CAD build for the part. Positions are in the model's coordinates, mm. A direction names the side the tool comes from. Coordinates: 2 decimals unless noted, no trailing zeros. Order: outer loops, then holes, each group sorted by start corner. A loop starts at its lowest first (then second) coordinate and runs counter-clockwise, first axis right, second up. Notation, with made-up numbers: M 50.5,35 L 97.5,35 A23 ccw 97.5,70 Z; hole C 8.5,42 d11. An arc over 180 degrees is marked long. Write item = value, one per line.
Autodesk Inventor part; units mm, degrees
ref_plane "YZ Plane" through (0, 0, 0) normal (1, 0, 0) x (0, 1, 0)
ref_plane "XZ Plane" through (0, 0, 0) normal (0, 1, 0) x (-1, 0, 0)
ref_plane "XY Plane" through (0, 0, 0) normal (0, 0, 1) x (1, 0, 0)
sketch "Sketch1" plane through (0, 0, 0) normal (0, 0, 1) x (1, 0, 0)
  circle A0 centre (0, 0) radius 15
  dimension "d0" = 30
extrude "Extrusion1" add sketch "Sketch1" along normal blind 10
sketch "Sketch2" plane through (0, 0, 10) normal (0, 0, 1) x (1, 0, 0)
  circle A0 centre (0, 0) radius 15
  circle A1 centre (0, 0) radius 7.5
  dimension "d3" = 15
extrude "Extrusion2" add sketch "Sketch2" along normal blind 43.2 contours A1
sketch "Sketch3" plane through (0, 0, 53.2) normal (0, 0, 1) x (1, 0, 0)
  circle A0 centre (0, 0) radius 7.5
  circle A1 centre (0, 0) radius 6.5
  dimension "d6" = 1
extrude "Extrusion3" cut sketch "Sketch3" against normal blind 1 contours A1
fillet "Fillet1" radius 2 1 edges at (-15, 0, 10)
chamfer "Chamfer1" distance 0.25 angle 45 1 edges at (-7.5, 0, 53.2)
chamfer "Chamfer2" distance 0.25 angle 45 1 edges at (-15, 0, 0)
properties part number "InfiniStix_066x"
(1) Pull direction X, two halves, no side cores. Call faces 1 (the face through (-7.493, -0.33, 31.174)), 2 (the face through (-3, 6, 53.2)), 3 (the face through (-5.158, -3.955, 52.707)): +X half, -X half, draft (parallel to the pull), parting line (faces both ways), or undercut.
Evaluation:
face_1 = parting line
face_2 = draft
face_3 = undercut
(2) Pin check, flat tips, straight feed: pin 1 Ø6 at (x, z) = (9, 38) entering from +Y; pin 2 Ø10 at (x, z) = (-7, 22.5) entering from -Y; pin 3 Ø6 at (x, z) = (9.5, 34) entering from -Y; pin 4 Ø1.5 at (x, z) = (-8.5, 34) entering from +Y. Stop position of each tip, or through.
Evaluation:
pin_1 = 4.5
pin_2 = -7.23
pin_3 = -3.74
pin_4 = through
(3) Slice it at A-A, the plane x = 0. Write the cut outline in (y, z), then the cut area to 3 significant figures.
Evaluation:
outline = M -15,0.25 L -14.75,0 L 14.75,0 L 15,0.25 L 15,8 A2 ccw 13,10 L 7.5,10 L 7.5,52.95 L 7.25,53.2 L 6.5,53.2 L 6.5,52.2 L -6.5,52.2 L -6.5,53.2 L -7.25,53.2 L -7.5,52.95 L -7.5,10 L -13,10 A2 ccw -15,8 Z
area = 933 mm²
(4) Wall check: line 1 (Y direction, x = 0, z = 52.55); line 2 (Y direction, x = -3.75, z = 37); line 3 (Z direction, x = 4, y = 6.75). Give the ranges that are in metal, low to high. Write a range as from..to.
Evaluation:
line_1 = -7.5..-6.5, 6.5..7.5
line_2 = -6.5..6.5
line_3 = 0..10
(5) Slice it at C-C, the plane z = 7. Write the cut outline in (x, y), then the cut area to 3 significant figures.
Evaluation:
outline = C 0,0 d30
area = 707 mm²
(6) Slice it at D-D, the plane z = 23.5. Write the cut outline in (x, y), then the cut area to 3 significant figures.
Evaluation:
outline = C 0,0 d15
area = 177 mm²
(7) Tool access for faces 4 (the face through (0, 0, 52.2)), 5 (the face through (-14.985, -0.66, 4.071)): list every direction of +Z, -Z, +X, -X, +Y, -Y with a clear straight run to the whole face (end or side of a thin tool).
Evaluation:
face_4 = +Z
face_5 = +Z, -Z
